from build123d import *

# Parameters (mm, degrees)
F0_W     = 26.1
F0_H     = 44.1
F0_W_2   = 22.1
F0_H_2   = 40.1
F1_DEPTH = 10
F2_R     = 7.5
F3_DEPTH = 10
F4_R     = 8.5
F4_R_2   = 7.5
F5_DEPTH = 1
F6_R     = 2
F7_R     = 2


with BuildPart() as f1:
    # F0 (on Top) → F1 (new body, symmetric)
    with BuildSketch(Plane.XY):
        Rectangle(F0_W, F0_H)
        Rectangle(F0_W_2, F0_H_2, mode=Mode.SUBTRACT)
    extrude(amount=F1_DEPTH, both=True)

    # F2 (on face) → F3 (cut)
    with BuildSketch(Plane.XZ.offset(22.05)):
        with Locations((0, 4)):
            Circle(F2_R)
    extrude(amount=-F3_DEPTH, mode=Mode.SUBTRACT)

    # F4 (on face) → F5 (cut)
    with BuildSketch(Plane.XZ.offset(22.05)):
        with Locations((0, 4)):
            Circle(F4_R)
        with Locations((0, 4)):
            Circle(F4_R_2, mode=Mode.SUBTRACT)
    extrude(amount=-F5_DEPTH, mode=Mode.SUBTRACT)

    # F6
    f6_edges = [f1.edges().sort_by_distance(p)[0] for p in [
        (-13.05, -22.05, 0),
        (13.05, -22.05, 0),
        (13.05, 22.05, 0),
        (-13.05, 22.05, 0),
    ]]
    fillet(f6_edges, radius=F6_R)

    # F7
    f7_edges = [f1.edges().sort_by_distance(p)[0] for p in [
        (-11.05, 20.05, 0),
        (11.05, 20.05, 0),
        (11.05, -20.05, 0),
        (-11.05, -20.05, 0),
    ]]
    fillet(f7_edges, radius=F7_R)


solid = f1.part
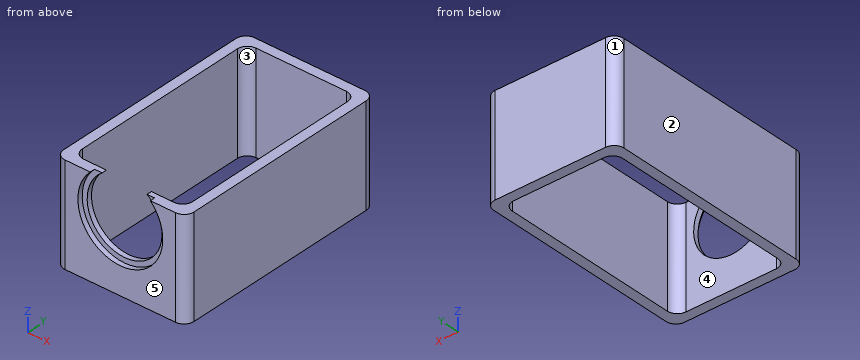
Input: part model. Units: mm. Frame: model coordinates. Face numbers are marked on the shaded views. A direction names the side the tool comes from. Give positions to 0.01 mm unless a question says otherwise; leave off trailing zeros. Write each loop counter-clockwise with the first axis right and the second up, starting at its lowest first coordinate (ties: lowest second). Pieces come first, ordered by that corner, then holes. Notation, with made-up numbers: (-20, -1.5) -> (37, -1.5) arc R21 ccw to (37, 28.5) -> close; hole circle Ø11 at (3, 21.5). An arc over 180 degrees is marked (long way). Use one line per item in the form item = value. Start each with the question number.
1) Set-up query: the marked faces 4 and 5. Return all of +Z, -Z, +X, -X, +Y, -Y with unobstructed straight access to the full face (end or side cutting, diameter ignored); none if empty.
2) Section query B-B on y = -15.5. Return the cut outline in (x, z), then the cut area to 3 significant figures.
3) Section query D-D on z = 4. Return the cut outline in (x, y).
4) Draft query along Y for the marked faces 1, 2 and 3. Return one class per face: pulls with the +Y half, pulls with the -Y half, needs draft (parallel to the pull), parting line crosses it, or undercut.
5) Ray query, probe 1 along X at (y, z) = (-5, -8.5); probe 2 along Y at (x, z) = (-8.5, 1.5); probe 3 along Z at (x, y) = (0, -20.55). Return the intervals inside material, ascending. Write a range as from..to.
6) Section query A-A on x = 0. Return the cut outline in (y, z), then the cut area to 3 significant figures.
7) Section query C-C on z = -7. Return the cut outline in (x, y), then the cut area to 3 significant figures.
Outcome:
q1.face_4 = +Z, -Z
q1.face_5 = +Z, -Z, +X, -X, -Y
q2.outline = (-13.05, -10) -> (-11.05, -10) -> (-11.05, 10) -> (-13.05, 10) -> close; (11.05, -10) -> (13.05, -10) -> (13.05, 10) -> (11.05, 10) -> close
q2.area = 80.0 mm^2
q3.outline = (-13.05, -20.05) arc R2 ccw to (-11.05, -22.05) -> (-8.5, -22.05) -> (-8.5, -21.05) -> (-7.5, -21.05) -> (-7.5, -20.05) -> (-9.05, -20.05) arc R2 cw to (-11.05, -18.05) -> (-11.05, 18.05) arc R2 cw to (-9.05, 20.05) -> (9.05, 20.05) arc R2 cw to (11.05, 18.05) -> (11.05, -18.05) arc R2 cw to (9.05, -20.05) -> (7.5, -20.05) -> (7.5, -21.05) -> (8.5, -21.05) -> (8.5, -22.05) -> (11.05, -22.05) arc R2 ccw to (13.05, -20.05) -> (13.05, 20.05) arc R2 ccw to (11.05, 22.05) -> (-11.05, 22.05) arc R2 ccw to (-13.05, 20.05) -> close
q4.face_1 = pulls with the +Y half
q4.face_2 = needs draft
q4.face_3 = undercut
q5.probe_1 = -13.05..-11.05, 11.05..13.05
q5.probe_2 = -22.05..-20.05, 20.05..22.05
q5.probe_3 = -10..-3.5
q6.outline = (-22.05, -10) -> (-20.05, -10) -> (-20.05, -3.5) -> (-21.05, -3.5) -> (-21.05, -4.5) -> (-22.05, -4.5) -> close; (20.05, -10) -> (22.05, -10) -> (22.05, 10) -> (20.05, 10) -> close
q6.area = 52.0 mm^2
q7.outline = (-13.05, -20.05) arc R2 ccw to (-11.05, -22.05) -> (11.05, -22.05) arc R2 ccw to (13.05, -20.05) -> (13.05, 20.05) arc R2 ccw to (11.05, 22.05) -> (-11.05, 22.05) arc R2 ccw to (-13.05, 20.05) -> close; hole (-11.05, -18.05) arc R2 ccw to (-9.05, -20.05) -> (9.05, -20.05) arc R2 ccw to (11.05, -18.05) -> (11.05, 18.05) arc R2 ccw to (9.05, 20.05) -> (-9.05, 20.05) arc R2 ccw to (-11.05, 18.05) -> close
q7.area = 265 mm^2
